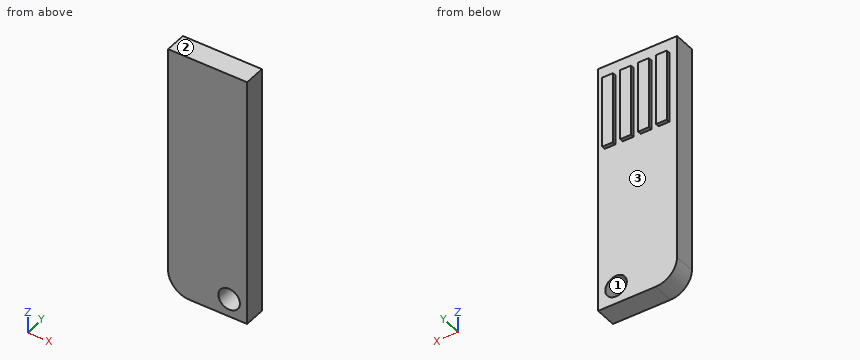
from build123d import *

# Parameters (mm, degrees)
SKETCH1_W           = 11
SKETCH1_H           = 35
BOSS_EXTRUDE1_DEPTH = 3
SKETCH2_R           = 1.5
CUT_EXTRUDE1_DEPTH  = 3
FILLET1_R           = 3
SKETCH3_W           = 1.5
SKETCH3_H           = 10
BOSS_EXTRUDE2_DEPTH = 0.5


with BuildPart() as part:
    # Sketch1 → Boss-Extrude1 (new body)
    with BuildSketch(Plane(origin=(0, 0, 0), x_dir=(1, 0, 0), z_dir=(0, 1, 0))):
        Rectangle(SKETCH1_W, SKETCH1_H)
    extrude(amount=BOSS_EXTRUDE1_DEPTH)

    # Sketch2 → Cut-Extrude1 (cut)
    with BuildSketch(Plane(origin=(0, 3, 0), x_dir=(1, 0, 0), z_dir=(0, 1, 0))):
        with Locations(Location((3, 15, 0), (0, 0, 270))):
            Circle(SKETCH2_R)
    extrude(amount=-CUT_EXTRUDE1_DEPTH, mode=Mode.SUBTRACT)

    # Fillet1
    fillet1_edges = [part.edges().sort_by_distance(p)[0] for p in [
        (-5.5, 1.5, -17.5),
    ]]
    fillet(fillet1_edges, radius=FILLET1_R)

    # Sketch3 → Boss-Extrude2 (add)
    with BuildSketch(Plane(origin=(0, 3, 0), x_dir=(1, 0, 0), z_dir=(0, 1, 0))):
        with Locations((-1.167481663, -10.550122249)):
            Rectangle(SKETCH3_W, SKETCH3_H)
        with Locations((-3.667481663, -10.550122249)):
            Rectangle(SKETCH3_W, SKETCH3_H)
        with Locations((1.332518337, -10.550122249)):
            Rectangle(SKETCH3_W, SKETCH3_H)
        with Locations((3.832518337, -10.550122249)):
            Rectangle(SKETCH3_W, SKETCH3_H)
    extrude(amount=BOSS_EXTRUDE2_DEPTH)


solid = part.part
Read the model definition and answer for the solid it produces. Units are mm, in the model's axes. Face numbers are marked on the shaded views. Give positions to 0.01 mm unless a question says otherwise; leave off trailing zeros. Write each loop counter-clockwise with the first axis right and the second up, starting at its lowest first coordinate (ties: lowest second). Pieces come first, ordered by that corner, then holes. Notation, with made-up numbers: (-24.75, 52) -> (-13.75, 52) arc R18 ccw to (-13.75, 72) -> close; hole circle Ø5 at (-15.5, 83). An arc over 180 degrees is marked (long way). Answer as a JSON object with one key per item and string values. Group by question number.
1) Consider L1, parallel to X at y = 3.3, z = 7.5; L2, parallel to Y at x = -0.75, z = 16; L3, parallel to X at y = 2.05, z = -15. Determine where each line is inside the solid, lowest interval first. Write a range as from..to.
2) Find section D-D (z = 13). Write down the section's boundary in (x, y), and give its area (3 significant figures).
3) The mould has two halves that part along Z. Classify the marked faces 1, 2 and 3: +Z half, -Z half, draft (parallel to the pull), parting line (faces both ways), or undercut.
4) Find section B-B (x = -1.25). Write down the section's boundary in (y, z), and give its area (3 significant figures).
5) Find section C-C (y = 1.8). Write down the section's boundary in (x, z), and give its area (3 significant figures).
6) Find section A-A (z = -15). Write down the section's boundary in (x, y), and give its area (3 significant figures).
7) This flat-tipped pin is pushed along its axis until it touches: P1, Ø2.5, axis at x = 3, z = -15, coming from the +Y side. Where does it stop, or does it pass through?
Values follow:
{
 "1": {"L1": "x = -4.42..-2.92, -1.92..-0.42, 0.58..2.08, 3.08..4.58", "L2": "y = 0..3", "L3": "x = -5.46..1.5, 4.5..5.5"},
 "2": {"outline": "(-5.5, 0) -> (5.5, 0) -> (5.5, 3) -> (4.58, 3) -> (4.58, 3.5) -> (3.08, 3.5) -> (3.08, 3) -> (2.08, 3) -> (2.08, 3.5) -> (0.58, 3.5) -> (0.58, 3) -> (-0.42, 3) -> (-0.42, 3.5) -> (-1.92, 3.5) -> (-1.92, 3) -> (-2.92, 3) -> (-2.92, 3.5) -> (-4.42, 3.5) -> (-4.42, 3) -> (-5.5, 3) -> close", "area": "36.0 mm2"},
 "3": {"face 1": "undercut", "face 2": "+Z half", "face 3": "draft"},
 "4": {"outline": "(0, -17.5) -> (3, -17.5) -> (3, 5.55) -> (3.5, 5.55) -> (3.5, 15.55) -> (3, 15.55) -> (3, 17.5) -> (0, 17.5) -> close", "area": "110 mm2"},
 "5": {"outline": "(-5.5, -14.5) arc R3 ccw to (-2.5, -17.5) -> (5.5, -17.5) -> (5.5, 17.5) -> (-5.5, 17.5) -> close; hole circle Ø3 at (3, -15)", "area": "376 mm2"},
 "6": {"outline": "(-5.46, 0) -> (1.5, 0) -> (1.5, 3) -> (-5.46, 3) -> close; (4.5, 0) -> (5.5, 0) -> (5.5, 3) -> (4.5, 3) -> close", "area": "23.9 mm2"},
 "7": {"P1": "passes through"}
}
